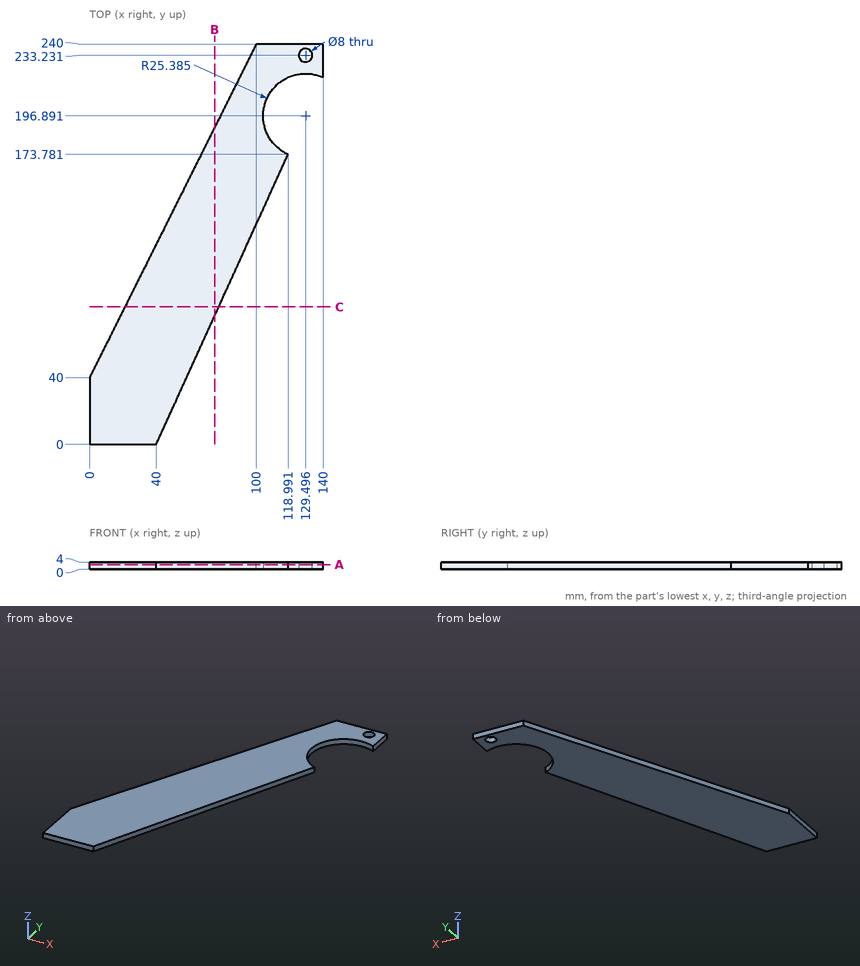
Could you check a few things on this drawing? It's one solid part, dimensions in mm from its lowest x, y, z. Coordinates: 2 decimals unless noted, no trailing zeros. Write each loop counter-clockwise with the first axis right and the second up, starting at its lowest first coordinate (ties: lowest second). Pieces come first, ordered by that corner, then holes.
Q1. For P1, Ø1.5, axis at y = 27, z = 1.5, coming from the +X side; P2, Ø5, axis at x = 129.5, y = 233.23, coming from the -Z side, each with a flat end and sliding along its axis, tell me the tip position at first contact or that it passes through.
Results found:
P1: stops at x = 52.61
P2: passes through
Q2. Imagine slicing it at B-B, the plane x = 75. List the corners of the cut face in (y, z) for me.
Results found:
outline: (77, 0) - (190, 0) - (190, 4) - (77, 4) - close
Q3. Please list where these lines run through material, in increasing order: L1, parallel to Y at x = 129.5, z = 1.5 (1 decimal); L2, parallel to Y at x = 111, z = 0.6 (1 decimal); L3, parallel to X at y = 64, z = 2.7.
Results found:
L1: y = 222.3 to 229.2, 237.2 to 240
L2: y = 156.2 to 179.5, 214.3 to 240
L3: x = 12 to 69.09
Q4. Imagine slicing it at A-A, the plane z = 2.65. List the corners of the cut face in (x, y) for me (1 decimal).
Results found:
outline: (0, 0) - (40, 0) - (119, 173.8) arc R25.4 cw to (140, 220) - (140, 240) - (100, 240) - (0, 40) - close; hole circle Ø8 at (129.5, 233.2)
Q5. Imagine slicing it at C-C, the plane y = 82.5. List the corners of the cut face in (x, z) for me, plus the area to 3 significant figures.
Results found:
outline: (21.25, 0) - (77.5, 0) - (77.5, 4) - (21.25, 4) - close
area: 225 mm2
